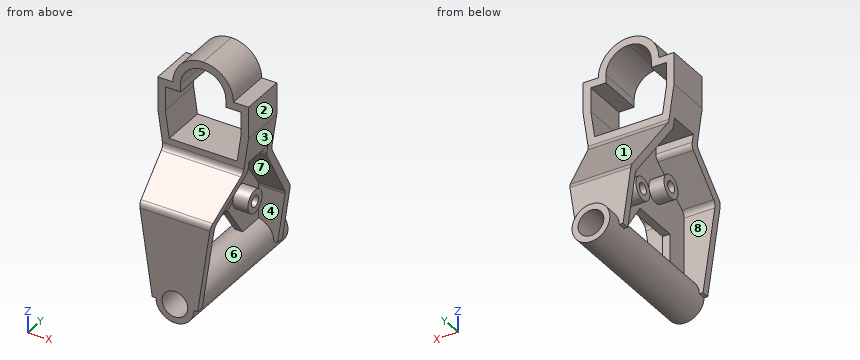
from build123d import *
from build123d.topology import SkipClean

# Parameters (mm, degrees)
BOSS_EXTRUDE1_DEPTH     = 60
CUT_EXTRUDE1_DEPTH      = 314.84709653
CUT_EXTRUDE2_REACH      = 290.725
CUT_EXTRUDE2_START      = 5
FILLET1_R               = 10
BOSS_EXTRUDE4_DEPTH     = 60
BOSS_EXTRUDE2_DEPTH     = 200
CUT_EXTRUDE3_DEPTH      = 306.982025616
CUT_EXTRUDE3_DEPTH_BACK = 306.982025616
SKETCH5_R               = 17
SKETCH6_R               = 15
BOSS_EXTRUDE3_DEPTH     = 20
CUT_EXTRUDE4_REACH      = 312.564
SKETCH7_R               = 7.5


with BuildPart() as part:
    # Sketch1 → Boss-Extrude1 (new body)
    with BuildSketch(Plane(origin=(0, 0, 0), x_dir=(0, 0, -1), z_dir=(1, 0, 0))):
        Polygon((0, 0), (0, 60), (90, 60), (175.688880405, 120), (250, 120), (250, 92.682857844), (180, 43.668330169), (180, -20), (250, -20), (250, -60), (132.012452293, -60), (90, 0), align=None)
    extrude(amount=BOSS_EXTRUDE1_DEPTH)

    # Sketch2 → Cut-Extrude1 (cut, through all)
    with BuildSketch(Plane(origin=(0, 120, 0), x_dir=(1, 0, 0), z_dir=(0, 1, 0))):
        Polygon((60, 42.034783703), (30, 250), (60, 250), align=None)
    extrude(amount=-CUT_EXTRUDE1_DEPTH, mode=Mode.SUBTRACT)

    # Cut-Extrude2: up to this plane
    cut_extrude2_end = Plane(origin=(60, -60, -42.034783703), z_dir=(-0.9897548850976273, 0, 0.1427769849288831))
    # Sketch4 → Cut-Extrude2 (cut, up to the surface)
    with BuildSketch(Plane(origin=(0, 0, 0), x_dir=(0, 0, -1), z_dir=(1, 0, 0)).offset(CUT_EXTRUDE2_START), mode=Mode.PRIVATE) as cut_extrude2_sk1:
        Polygon((80, 50), (80, 10), (95.205670506, 10), (137.218122798, -50), (250, -50), (250, 110), (178.841868293, 110), (93.152987889, 50), align=None)
    cut_extrude2_tool1 = split(extrude(cut_extrude2_sk1.sketch, amount=CUT_EXTRUDE2_REACH, mode=Mode.PRIVATE), bisect_by=cut_extrude2_end, keep=Keep.BOTH, mode=Mode.PRIVATE)
    add(cut_extrude2_tool1.solids().sort_by_distance((5, 26.655834, -179.495855))[0], mode=Mode.SUBTRACT)

    # Fillet1
    fillet1_edges = [part.edges().sort_by_distance(p)[0] for p in [
        (26.540391431, 60, -90),
        (20.359871299, 120, -175.688880405),
        (23.510140528, -60, -132.012452293),
        (26.540391431, 0, -90),
        (28.66491971, 10, -95.205670506),
        (25.634668807, -50, -137.218122798),
        (22.632454334, 110, -178.841868293),
        (28.812974465, 50, -93.152987889),
    ]]
    fillet(fillet1_edges, radius=FILLET1_R)

    # Sketch8 → Boss-Extrude4 (add)
    with BuildSketch(Plane(origin=(0, 60, 0), x_dir=(1, 0, 0), z_dir=(0, 1, 0))):
        with BuildLine():
            Line((0, 0), (0, -40))
            ThreePointArc((0, -40), (28.284271247, -28.284271247), (40, 0))
            Line((40, 0), (0, 0))
        make_face()
    extrude(amount=-BOSS_EXTRUDE4_DEPTH)

    # Sketch3 → Boss-Extrude2 (add)
    with BuildSketch(Plane.XZ.offset(60)):
        with BuildLine():
            Line((0, -275), (0, -225))
            ThreePointArc((0, -225), (25, -250), (0, -275))
        make_face()
    extrude(amount=-BOSS_EXTRUDE2_DEPTH)

    # Sketch5 → Cut-Extrude3 (cut, two sides: drawn at the far end of the back side and taken through both)
    with BuildSketch(Plane(origin=(0, 60, 0), x_dir=(1, 0, 0), z_dir=(0, 1, 0)).offset(-CUT_EXTRUDE3_DEPTH_BACK)):
        with Locations((0, 250)):
            Circle(SKETCH5_R)
        with BuildLine():
            Line((40, 10), (30, 10))
            Line((30, 10), (30, 0))
            ThreePointArc((30, 0), (21.213203436, -21.213203436), (0, -30))
            Line((0, -30), (0, 76.847012111))
            Line((0, 76.847012111), (44.874654082, 76.847012111))
            Line((44.874654082, 76.847012111), (50, 41.317223033))
            Line((50, 41.317223033), (50, 10))
            Line((50, 10), (40, 10))
        make_face()
    extrude(amount=CUT_EXTRUDE3_DEPTH + CUT_EXTRUDE3_DEPTH_BACK, mode=Mode.SUBTRACT)

    # Sketch6 → Boss-Extrude3 (add)
    with BuildSketch(Plane(origin=(5, 0, 0), x_dir=(0, 0, -1), z_dir=(1, 0, 0))):
        with Locations((175, 70)):
            Circle(SKETCH6_R)
        with Locations((140, 10)):
            Circle(SKETCH6_R)
    extrude(amount=BOSS_EXTRUDE3_DEPTH)

    # Sketch7 → Cut-Extrude4 (cut, up to next)
    with BuildSketch(Plane(origin=(25, 0, 0), x_dir=(0, 0, -1), z_dir=(1, 0, 0)), mode=Mode.PRIVATE) as cut_extrude4_sk1:
        with Locations((140, 10)):
            Circle(SKETCH7_R)
    cut_extrude4_tool1 = extrude(cut_extrude4_sk1.sketch, amount=-CUT_EXTRUDE4_REACH, mode=Mode.PRIVATE) & part.part
    # Sketch7 → Cut-Extrude4 (cut, up to next)
    with BuildSketch(Plane(origin=(25, 0, 0), x_dir=(0, 0, -1), z_dir=(1, 0, 0)), mode=Mode.PRIVATE) as cut_extrude4_sk2:
        with Locations((175, 70)):
            Circle(SKETCH7_R)
    cut_extrude4_tool2 = extrude(cut_extrude4_sk2.sketch, amount=-CUT_EXTRUDE4_REACH, mode=Mode.PRIVATE) & part.part
    add(cut_extrude4_tool1.solids().sort_by_distance((25, 10, -140))[0], mode=Mode.SUBTRACT)
    add(cut_extrude4_tool2.solids().sort_by_distance((25, 70, -175))[0], mode=Mode.SUBTRACT)

    # Mirror2: part across plane


with BuildPart() as part_1:
    with SkipClean():  # the faces are left unmerged after this step: merging them gives an invalid solid
        add(part.part)
        add(part.part.mirror(Plane.ZY))


solid = part_1.part
Geometry check sheet. Reference: the model listing, model coordinates, mm. Face numbers are marked on the shaded views. A direction names the side the tool comes from. Round coordinates to 2 decimals unless told otherwise and drop trailing zeros. Order: outer loops, then holes, each group sorted by start corner. A loop starts at its lowest first (then second) coordinate and runs counter-clockwise, first axis right, second up. Notation, with made-up numbers: M 65,28.5 L 82,28.5 A13 ccw 82,42.5 Z; hole C -24.5,-26.75 d10. An arc over 180 degrees is marked long. Answer in a Markdown table with one row per item. Add a question column.
Item 1: Material ranges on L1, parallel to Z at x = 9, y = -36; L2, parallel to Z at x = 0, y = 44; L3, parallel to Z at x = 0, y = 5, recorded low to high. Write a range as [from, to].
Item 2: Depth check by flat-ended pin: pin 1 Ø1 at (x, y) = (-4.5, -10.5) entering from -Z; pin 2 Ø2 at (y, z) = (42.5, -157.5) entering from -X; pin 3 Ø16 at (x, y) = (44, 26.5) entering from -Z. Enter the tip coordinate at first touch or a pass-through.
Item 3: Sectioned sample at D-D, the plane x = 9. State how many separate pieces and enclosed holes the cut face has, plus the area to 3 significant figures.
Item 4: Sectioned sample at A-A, the plane y = -9.5. Enter the section's corners in (x, z).
Item 5: Sectioned sample at B-B, the plane y = 70. Enter the section's corners in (x, z), plus the area to 3 significant figures.
Item 6: Set-up check for the marked faces 5, 6, 7 and 8: record each of +Z, -Z, +X, -X, +Y, -Y from which the full face is reachable in a straight line by a thin tool's end or side.
Item 7: Sectioned sample at C-C, the plane z = -236.5. Enter the section's corners in (x, y), plus the area to 3 significant figures.
Item 8: Draft check along Z on the marked faces 1, 2, 3 and 4. Enter one of: released by +Z, released by -Z, zero draft, split by the parting line, or undercut.
Filled in:
| question | item | result |
|---|---|---|
| 1 | L1 | z = [-273.32, -264.42], [-235.58, -226.68], [-127.42, -115.21] |
| 1 | L2 | z = [-275, -267], [-233, -225], [-180.47, -76.85], [30, 40] |
| 1 | L3 | z = [-275, -267], [-233, -225], [-180, -145.59], [-134.41, -76.85], [30, 40] |
| 2 | pin 1 | stops at z = -274.68 |
| 2 | pin 2 | stops at x = -5 |
| 2 | pin 3 | stops at z = -80 |
| 3 | separate pieces | 5 |
| 3 | enclosed holes | 3 |
| 3 | area | 8,870 mm² |
| 4 | outline | M -52.12,-96.65 L -50.36,-108.86 L -5,-108.86 L -5,-180 L 5,-180 L 5,-108.86 L 50.36,-108.86 L 52.12,-96.65 Z; C 0,-250 d50; hole C 0,-250 d34 |
| 5 | outline | M -51.02,-104.28 L -48.51,-121.72 L -5,-121.72 L -5,-160 L -25,-160 L -25,-167.5 L 25,-167.5 L 25,-160 L 5,-160 L 5,-121.72 L 48.51,-121.72 L 51.02,-104.28 Z; C 0,-250 d50; M -25,-190 L -5,-190 L -5,-217.61 L 5,-217.61 L 5,-190 L 25,-190 L 25,-182.5 L -25,-182.5 Z; hole C 0,-250 d34 |
| 5 | area | 4,200 mm² |
| 6 | face 5 | +Y, -Y |
| 6 | face 6 | none |
| 6 | face 7 | +X |
| 6 | face 8 | -X |
| 7 | outline | M -31.95,-60 L -10.33,-60 L -10.33,140 L -21.04,140 L -21.04,120 L -31.95,120 L -31.95,110 L -21.04,110 L -21.04,-50 L -31.95,-50 Z; M 10.33,-60 L 31.95,-60 L 31.95,-50 L 21.04,-50 L 21.04,110 L 31.95,110 L 31.95,120 L 21.04,120 L 21.04,140 L 10.33,140 Z |
| 7 | area | 4,720 mm² |
| 8 | face 1 | released by +Z |
| 8 | face 2 | zero draft |
| 8 | face 3 | released by -Z |
| 8 | face 4 | undercut |
